from build123d import *

# Parameters (mm, degrees)
BOSS_EXTRUDE1_DEPTH                               = 450
FRONTSIDEHOLES_SKETCH3_R                          = 1.5875
FRONTSIDEHOLES_SKETCH3_R_2                        = 2
FRONTSIDEHOLES_CUT_EXTRUDE1_DEPTH                 = 3.175
LEFTSIDEHOLES_SKETCH4_R                           = 1.5875
LEFTSIDEHOLES_CUT_EXTRUDE2_DEPTH                  = 3.175
CSK_FOR_6_FLAT_HEAD_MACHINE_SCREW_100_D           = 3.7973
CSK_FOR_6_FLAT_HEAD_MACHINE_SCREW_100_CSINK_D     = 7.0866
CSK_FOR_6_FLAT_HEAD_MACHINE_SCREW_100_CSINK_ANGLE = 100
CSK_FOR_6_FLAT_HEAD_MACHINE_SCREW_2_D             = 3.7973
CSK_FOR_6_FLAT_HEAD_MACHINE_SCREW_2_CSINK_D       = 7.0866
CSK_FOR_6_FLAT_HEAD_MACHINE_SCREW_2_CSINK_ANGLE   = 100


with BuildPart() as part:
    # Sketch2 → Boss-Extrude1 (new body)
    with BuildSketch(Plane(origin=(0, 0, 0), x_dir=(1, 0, 0), z_dir=(0, 1, 0))):
        Polygon((0, 31.75), (3.175, 31.75), (3.175, 3.175), (31.75, 3.175), (31.75, 0), (0, 0), align=None)
    extrude(amount=BOSS_EXTRUDE1_DEPTH)

    # FrontSideHoles-Sketch3 → FrontSideHoles-Cut-Extrude1 (cut)
    with BuildSketch(Plane.XY):
        with Locations((19.05, 81.1125)):
            Circle(FRONTSIDEHOLES_SKETCH3_R)
        with Locations((14.2875, 87.4625)):
            Circle(FRONTSIDEHOLES_SKETCH3_R)
        with Locations((23.8125, 87.4625)):
            Circle(FRONTSIDEHOLES_SKETCH3_R)
        with Locations((14.2875, 438.8875)):
            Circle(FRONTSIDEHOLES_SKETCH3_R)
        with Locations((23.8125, 438.8875)):
            Circle(FRONTSIDEHOLES_SKETCH3_R)
        with Locations((19.05, 426.1875)):
            Circle(FRONTSIDEHOLES_SKETCH3_R)
        with Locations((14.2875, 354.18487)):
            Circle(FRONTSIDEHOLES_SKETCH3_R_2)
        with Locations((14.2875, 313.98487)):
            Circle(FRONTSIDEHOLES_SKETCH3_R_2)
        with Locations((14.2875, 260)):
            Circle(FRONTSIDEHOLES_SKETCH3_R)
        with Locations((14.2875, 165)):
            Circle(FRONTSIDEHOLES_SKETCH3_R)
        with Locations((23.8125, 7.9375)):
            Circle(FRONTSIDEHOLES_SKETCH3_R)
    extrude(amount=-FRONTSIDEHOLES_CUT_EXTRUDE1_DEPTH, mode=Mode.SUBTRACT)

    # LeftSideHoles-Sketch4 → LeftSideHoles-Cut-Extrude2 (cut)
    with BuildSketch(Plane.ZY):
        with Locations((-23.8125, 81.1125)):
            Circle(LEFTSIDEHOLES_SKETCH4_R)
        with Locations((-14.2875, 81.1125)):
            Circle(LEFTSIDEHOLES_SKETCH4_R)
        with Locations((-19.05, 87.4625)):
            Circle(LEFTSIDEHOLES_SKETCH4_R)
        with Locations((-19.05, 438.8875)):
            Circle(LEFTSIDEHOLES_SKETCH4_R)
        with Locations((-23.8125, 426.1875)):
            Circle(LEFTSIDEHOLES_SKETCH4_R)
        with Locations((-14.2875, 426.1875)):
            Circle(LEFTSIDEHOLES_SKETCH4_R)
        with Locations((-23.8125, 341.24737)):
            Circle(LEFTSIDEHOLES_SKETCH4_R)
        with Locations((-14.2875, 341.24737)):
            Circle(LEFTSIDEHOLES_SKETCH4_R)
        with Locations((-23.8125, 306.32237)):
            Circle(LEFTSIDEHOLES_SKETCH4_R)
        with Locations((-14.2875, 306.32237)):
            Circle(LEFTSIDEHOLES_SKETCH4_R)
        with Locations((-23.8125, 7.9375)):
            Circle(LEFTSIDEHOLES_SKETCH4_R)
        with Locations((-14.2875, 165)):
            Circle(LEFTSIDEHOLES_SKETCH4_R)
        with Locations((-14.2875, 260)):
            Circle(LEFTSIDEHOLES_SKETCH4_R)
        with Locations((-14.2875, 355)):
            Circle(LEFTSIDEHOLES_SKETCH4_R)
    extrude(amount=-LEFTSIDEHOLES_CUT_EXTRUDE2_DEPTH, mode=Mode.SUBTRACT)

    # CSK for _6 Flat Head Machine Screw _100 (through all)
    with Locations(Plane.XY):
        with Locations((14.2875, 87.4625), (19.05, 81.1125), (23.8125, 87.4625), (19.05, 426.1875), (14.2875, 438.8875), (23.8125, 438.8875)):
            CounterSinkHole(CSK_FOR_6_FLAT_HEAD_MACHINE_SCREW_100_D / 2, CSK_FOR_6_FLAT_HEAD_MACHINE_SCREW_100_CSINK_D / 2, counter_sink_angle=CSK_FOR_6_FLAT_HEAD_MACHINE_SCREW_100_CSINK_ANGLE)

    # CSK for _6 Flat Head Machine Screw _ 2 (through all)
    with Locations(Plane.ZY):
        with Locations((-19.05, 87.4625), (-23.8125, 81.1125), (-14.2875, 81.1125), (-23.8125, 341.24737), (-14.2875, 341.24737), (-14.2875, 306.32237), (-23.8125, 306.32237), (-23.8125, 426.1875), (-14.2875, 426.1875), (-19.05, 438.8875)):
            CounterSinkHole(CSK_FOR_6_FLAT_HEAD_MACHINE_SCREW_2_D / 2, CSK_FOR_6_FLAT_HEAD_MACHINE_SCREW_2_CSINK_D / 2, counter_sink_angle=CSK_FOR_6_FLAT_HEAD_MACHINE_SCREW_2_CSINK_ANGLE)


solid = part.part
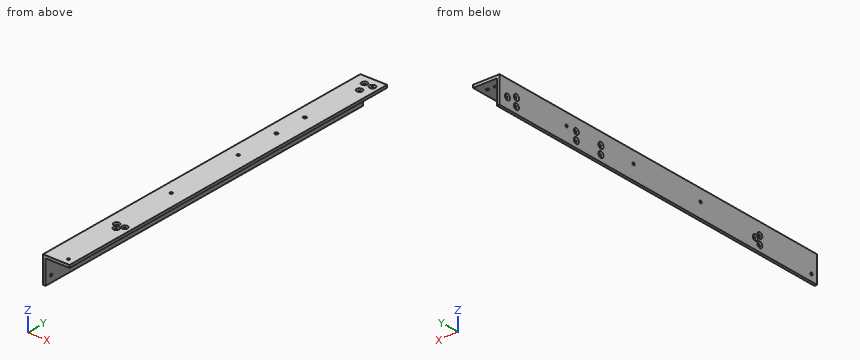
Input: part model. Units: mm. Frame: model coordinates. Give positions to 0.01 mm unless a question says otherwise; leave off trailing zeros. Order: outer loops, then holes, each group sorted by start corner. A loop starts at its lowest first (then second) coordinate and runs counter-clockwise, first axis right, second up. Notation, with made-up numbers: (89, 60.5) - (144, 60.5) arc R10 cw to (144, 76.5) - close; hole circle Ø6 at (33.5, -39.5). An arc over 180 degrees is marked (long way). Write each question's results on one line, items separated by ' | '.
Item 1: Contact query for flat-ended pins moving along their axis: pin 1 Ø1.5 at (y, z) = (265.5, -12) entering from +X (3 decimals); pin 2 Ø5 at (y, z) = (81.11, -23.81) entering from -X; pin 3 Ø4.5 at (x, y) = (14.29, 87.46) entering from +Z. Output: stop coordinate, or through.
A:
pin 1: stops at x = 3.175 | pin 2: stops at x = 0.87 | pin 3: stops at z = -1.08
Item 2: Material intervals for line 1 along Y through (x, z) = (2.5, -19.05); line 2 along Y through (x, z) = (19.05, -2.4); line 3 along Y through (x, z) = (23, -0.5), sorted ascending.
A:
line 1: y = 0 to 85.56, 89.36 to 436.99, 440.79 to 450 | line 2: y = 0 to 79.21, 83.01 to 424.29, 428.09 to 450 | line 3: y = 0 to 6.57, 9.3 to 84.63, 90.3 to 436.05, 441.72 to 450
Item 3: Section A-A (y = 417.5). Return loops of the section in (x, z) (3 decimals), and give its area (3 significant figures).
A:
outline: (0, -31.75) - (3.175, -31.75) - (3.175, -3.175) - (31.75, -3.175) - (31.75, 0) - (0, 0) - close | area: 192 mm^2
